```python
from build123d import *

# Parameters (mm, degrees)
SKETCH1_R            = 9.525
BOSS_EXTRUDE1_DEPTH  = 15.875
SKETCH1_3_W          = 58.7375
SKETCH1_3_H          = 9.525
SKETCH1_3_R          = 9.525
BOSS_EXTRUDE2_DEPTH  = 22.225
BOSS_EXTRUDE6_START  = 22.225
SKETCH1_7_R          = 9.525
SKETCH1_7_W          = 58.7375
SKETCH1_7_H          = 9.525
SKETCH1_7_W_2        = 9.525
BOSS_EXTRUDE6_DEPTH  = 9.525
BOSS_EXTRUDE8_START  = 15.875
SKETCH1_9_W          = 9.525
SKETCH1_9_H          = 9.525
BOSS_EXTRUDE8_DEPTH  = 9.525
BOSS_EXTRUDE10_START = 15.875
BOSS_EXTRUDE10_DEPTH = 9.525
CUT_EXTRUDE1_DEPTH   = 153.513472698
FILLET1_R            = 2.54


with BuildPart() as part:
    # Sketch1 → Boss-Extrude1 (new, symmetric)
    with BuildSketch(Plane.XY):
        with BuildLine():
            Line((0, -19.05), (95.25, -19.05))
            ThreePointArc((95.25, -19.05), (107.598173959, -28.781397654), (101.022727273, -43.062188994))
            ThreePointArc((101.022727273, -43.062188994), (98.945429127, -49.469032594), (105.352272727, -51.546330739))
            ThreePointArc((105.352272727, -51.546330739), (116.859304428, -26.554945895), (95.25, -9.525))
            Line((95.25, -9.525), (19.05, -9.525))
            Line((19.05, -9.525), (19.05, 0))
            ThreePointArc((19.05, 0), (-13.470384182, 13.470384182), (0, -19.05))
        make_face()
        Circle(SKETCH1_R, mode=Mode.SUBTRACT)
    extrude(amount=BOSS_EXTRUDE1_DEPTH, both=True)

    # Sketch1_3 → Boss-Extrude2 (add, symmetric)
    with BuildSketch(Plane.XY):
        with Locations((48.41875, -14.2875)):
            Rectangle(SKETCH1_3_W, SKETCH1_3_H)
        with BuildLine():
            ThreePointArc((-3.973521059, 18.63098576), (-18.944956832, -1.997776423), (0, -19.05))
            Line((0, -19.05), (19.05, -19.05))
            Line((19.05, -19.05), (19.05, -9.525))
            Line((19.05, -9.525), (19.05, 0))
            ThreePointArc((19.05, 0), (11.983466189, 14.808748701), (-3.973521059, 18.63098576))
        make_face()
        Circle(SKETCH1_3_R, mode=Mode.SUBTRACT)
    extrude(amount=BOSS_EXTRUDE2_DEPTH, both=True)

    # Sketch1_7 → Boss-Extrude6 (add)
    with BuildSketch(Plane.XY.offset(BOSS_EXTRUDE6_START)):
        with BuildLine():
            ThreePointArc((-3.973521059, 18.63098576), (-18.944956832, -1.997776423), (0, -19.05))
            Line((0, -19.05), (19.05, -19.05))
            Line((19.05, -19.05), (19.05, -9.525))
            Line((19.05, -9.525), (19.05, 0))
            ThreePointArc((19.05, 0), (11.983466189, 14.808748701), (-3.973521059, 18.63098576))
        make_face()
        Circle(SKETCH1_7_R, mode=Mode.SUBTRACT)
        with Locations((48.41875, -14.2875)):
            Rectangle(SKETCH1_7_W, SKETCH1_7_H)
        with BuildLine():
            Line((77.7875, 36.068556867), (-3.973521059, 18.63098576))
            ThreePointArc((-3.973521059, 18.63098576), (11.983466189, 14.808748701), (19.05, 0))
            Line((19.05, 0), (19.05, -9.525))
            Line((19.05, -9.525), (77.7875, -9.525))
            Line((77.7875, -9.525), (77.7875, 36.068556867))
        make_face()
        Polygon((87.3125, 38.1), (77.7875, 36.068556867), (77.7875, -9.525), (87.3125, -9.525), align=None)
        with Locations((82.55, -14.2875)):
            Rectangle(SKETCH1_7_W_2, SKETCH1_7_H)
    boss_extrude6 = extrude(amount=BOSS_EXTRUDE6_DEPTH)

    # Sketch1_9 → Boss-Extrude8 (add)
    with BuildSketch(Plane.XY.offset(BOSS_EXTRUDE8_START)):
        Polygon((87.3125, 38.1), (77.7875, 36.068556867), (77.7875, -9.525), (87.3125, -9.525), align=None)
        with Locations((82.55, -14.2875)):
            Rectangle(SKETCH1_9_W, SKETCH1_9_H)
    boss_extrude8 = extrude(amount=BOSS_EXTRUDE8_DEPTH)

    # Sketch1_10 → Boss-Extrude10 (add)
    with BuildSketch(Plane.XY.offset(BOSS_EXTRUDE10_START)):
        with BuildLine():
            Line((87.3125, -19.05), (95.25, -19.05))
            ThreePointArc((95.25, -19.05), (107.598173959, -28.781397654), (101.022727273, -43.062188994))
            ThreePointArc((101.022727273, -43.062188994), (98.945429127, -49.469032594), (105.352272727, -51.546330739))
            ThreePointArc((105.352272727, -51.546330739), (104.635512697, -51.896036246), (103.906667348, -52.219800571))
            ThreePointArc((103.906667348, -52.219800571), (138.961341357, -31.495116154), (127.958197617, 7.712963905))
            Line((127.958197617, 7.712963905), (87.3125, 38.1))
            Line((87.3125, 38.1), (87.3125, -19.05))
        make_face()
    boss_extrude10 = extrude(amount=BOSS_EXTRUDE10_DEPTH)

    # Mirror1: Boss-Extrude6, Boss-Extrude8, Boss-Extrude10 across plane
    add(boss_extrude6.mirror(Plane.XY))
    add(boss_extrude8.mirror(Plane.XY))
    add(boss_extrude10.mirror(Plane.XY))

    # Sketch2 → Cut-Extrude1 (cut, through all)
    with BuildSketch(Plane(origin=(0, -9.525, 0), x_dir=(1, 0, 0), z_dir=(0, 1, 0))):
        with BuildLine():
            Line((28.575, 15.875), (28.575, 0))
            Line((28.575, 0), (73.303122601, 0))
            ThreePointArc((73.303122601, 0), (75.787487527, 5.037793711), (81.296623537, 6.133628997))
            Line((81.296623537, 6.133628997), (46.556347172, 15.442257994))
            ThreePointArc((46.556347172, 15.442257994), (44.92702794, 15.766349739), (43.269345299, 15.875))
            Line((43.269345299, 15.875), (28.575, 15.875))
        make_face()
        with BuildLine():
            Line((28.575, 0), (28.575, -15.875))
            Line((28.575, -15.875), (43.269345299, -15.875))
            ThreePointArc((43.269345299, -15.875), (44.92702794, -15.766349739), (46.556347172, -15.442257994))
            Line((46.556347172, -15.442257994), (81.296623537, -6.133628997))
            ThreePointArc((81.296623537, -6.133628997), (75.787487527, -5.037793711), (73.303122601, 0))
            Line((73.303122601, 0), (28.575, 0))
        make_face()
        with BuildLine():
            ThreePointArc((81.296623537, 6.133628997), (75.787487527, 5.037793711), (73.303122601, 0))
            Line((73.303122601, 0), (86.003122601, 0))
            ThreePointArc((86.003122601, 0), (84.690916312, 3.865635074), (81.296623537, 6.133628997))
        make_face()
        with BuildLine():
            Line((86.003122601, 0), (73.303122601, 0))
            ThreePointArc((73.303122601, 0), (75.787487527, -5.037793711), (81.296623537, -6.133628997))
            ThreePointArc((81.296623537, -6.133628997), (84.690916312, -3.865635074), (86.003122601, 0))
        make_face()
    extrude(amount=-CUT_EXTRUDE1_DEPTH, mode=Mode.SUBTRACT)

    # Fillet1
    fillet1_edges = [part.edges().sort_by_distance(p)[0] for p in [
        (87.3125, 9.525, 25.4),
        (87.3125, 9.525, -31.75),
        (87.3125, 9.525, -25.4),
        (87.3125, 9.525, 31.75),
    ]]
    fillet(fillet1_edges, radius=FILLET1_R)


solid = part.part
```
Source: CAD feature listing. Evaluate the final solid. Frame: model axes, mm. A direction names the side the tool comes from. Give positions to 0.01 mm unless a question says otherwise; leave off trailing zeros. Loops run counter-clockwise (first coordinate to the right, second up) from the corner with the lowest first, then second, coordinate; pieces in that order, holes last. Notation, with made-up numbers: (2.25, -22.5) -> (40.25, -22.5) arc R28 ccw to (40.25, 11.5) -> close; hole circle Ø3 at (1.5, -23). An arc over 180 degrees is marked (long way). Put each result on its own line as item: value. Start each with the question number.
1) Reachability of faces 1 (the face through (116.953, -26.96, 0.222)), 2 (the face through (26, -19.05, 0)), 3 (the face through (44.9, -14.22, 15.77)), 4 (the face through (77.788, 14, 19)) from +Z, -Z, +X, -X, +Y, -Y: full face, straight path, thin tool, end or side. Return the list, or none.
2) Draft query along Y for faces 5 (the face through (98.9, -49.38, 0.36)), 6 (the face through (138.73, -32.06, 20.57)), 7 (the face through (19.05, -5, 0)). Return one class per face: released by +Y, released by -Y, zero draft, split by the parting line, or undercut.
3) Material intervals for probe 1 along Y at (x, z) = (0, -2.75) (3 decimals); probe 2 along Z at (x, y) = (127, -35) (3 decimals); probe 3 along Y at (x, z) = (-0.5, 19.5), sorted ascending.
4) Contact query for flat-ended pins moving along their axis: P1, Ø3, axis at y = -4, z = -3.5, coming from the +X side; P2, Ø1, axis at y = -7.5, z = -17, coming from the +X side; P3, Ø5, axis at y = 10.5, z = -20.5, coming from the -X side. Output: stop coordinate, or through.
5) Cut plane A-A (z = 11). State how many separate pieces and enclosed holes the cut face has, then the cut area to 3 significant figures.
6) Cut plane B-B (x = 35). Return loops of the section in (y, z) (3 decimals), then the cut area to 3 significant figures.
7) Cut plane D-D (x = 17). Return loops of the section in (y, z) (3 decimals).
Results are:
1. face 1: +X
1. face 2: +Z, -Z, -X, -Y
1. face 3: +Y, -Y
1. face 4: +Y
2. face 5: undercut
2. face 6: split by the parting line
2. face 7: zero draft
3. probe 1: y = -19.05 to -9.525, 9.525 to 19.05
3. probe 2: z = -25.4 to -15.875, 15.875 to 25.4
3. probe 3: y = -19.04 to -9.51, 9.51 to 19.04
4. P1: stops at x = 19.05
4. P2: stops at x = 139.49
4. P3: stops at x = -17.29
5. separate pieces: 2
5. enclosed holes: 1
5. area: 1,810 mm2
6. outline: (-19.05, -31.75) -> (26.943, -31.75) -> (26.943, -22.225) -> (-9.525, -22.225) -> (-9.525, -15.875) -> (-19.05, -15.875) -> close; (-19.05, 15.875) -> (-9.525, 15.875) -> (-9.525, 22.225) -> (26.943, 22.225) -> (26.943, 31.75) -> (-19.05, 31.75) -> close
6. area: 997 mm2
7. outline: (-19.05, -31.75) -> (23.104, -31.75) -> (23.104, -22.225) -> (8.597, -22.225) -> (8.597, 22.225) -> (23.104, 22.225) -> (23.104, 31.75) -> (-19.05, 31.75) -> close
